from build123d import *

# Parameters (mm, degrees)
SKETCH1_R           = 5.25
BOSS_EXTRUDE1_DEPTH = 8
SKETCH2_R           = 4
BOSS_EXTRUDE2_DEPTH = 2
FILLET2_R           = 1.2
FILLET3_R           = 1.2


with BuildPart() as part:
    # Sketch1 → Boss-Extrude1 (new body)
    with BuildSketch(Plane.XY):
        with Locations((0, 174.50846383)):
            Circle(SKETCH1_R)
    extrude(amount=BOSS_EXTRUDE1_DEPTH)

    # Sketch2 → Boss-Extrude2 (add)
    with BuildSketch(Plane.XY.offset(8)):
        with Locations((0.038551533, 174.508746935)):
            Circle(SKETCH2_R)
    extrude(amount=BOSS_EXTRUDE2_DEPTH)

    # Fillet2
    fillet2_edges = [part.edges().sort_by_distance(p)[0] for p in [
        (-3.961448467, 174.508746935, 8),
    ]]
    fillet(fillet2_edges, radius=FILLET2_R)

    # Fillet3
    fillet3_edges = [part.edges().sort_by_distance(p)[0] for p in [
        (-3.961448467, 174.508746935, 10),
    ]]
    fillet(fillet3_edges, radius=FILLET3_R)


solid = part.part
CAD build for the part. Positions are in the model's coordinates, mm. Round coordinates to 2 decimals unless told otherwise and drop trailing zeros. Order: outer loops, then holes, each group sorted by start corner. A loop starts at its lowest first (then second) coordinate and runs counter-clockwise, first axis right, second up. Notation, with made-up numbers: (-24.75, 39.25) -> (14.25, 39.25) arc R15 cw to (14.25, 57.25) -> close; hole circle Ø10 at (-34, -11.5). An arc over 180 degrees is marked (long way). Write item = value, one per line. Start each with the question number.
(1) Pin check, flat tips, straight feed: P1, Ø2, axis at x = 3, z = 5, coming from the +Y side; P2, Ø1.5, axis at y = 178, z = 8, coming from the +X side. Stop position of each tip, or through.
(2) Cut at A-A, the plane z = 7. List the corners of the cut face in (x, y), then the cut area to 3 significant figures.
(3) Probe line 1 (Y direction, x = -2.5, z = 4); line 2 (Z direction, x = -4.25, y = 174.5); line 3 (Z direction, x = 0.75, y = 171). List the from-to ranges inside material, lowest first. Write a range as [from, to].
Model answer:
q1.P1 = 179.36
q1.P2 = 4.48
q2.outline = circle Ø10.5 at (0, 174.51)
q2.area = 86.6 mm2
q3.line_1 = [169.89, 179.13]
q3.line_2 = [0, 8.42]
q3.line_3 = [0, 9.74]
